from build123d import *

# Parameters (mm, degrees)
TAP_DRILL_FOR_M5_TAP1_D     = 4.1
TAP_DRILL_FOR_M5_TAP1_DEPTH = 5.5
TAP_DRILL_FOR_M5_TAP1_TIP   = 1.231764269
SKETCH5_R                   = 1.75
CUT_EXTRUDE1_DEPTH          = 29.8


with BuildPart() as part:
    # Sketch2 → Revolve4 (revolve)
    with BuildSketch(Plane.XY):
        Polygon((292.362244726, 80.31885353), (304.262244726, 80.31885353), (304.262244726, 80.06885353), (307.762244726, 80.06885353), (307.762244726, 76.84385353), (284.762244726, 76.84385353), (284.762244726, 79.76885353), (287.762244726, 79.76885353), (287.762244726, 79.49385353), (288.762244726, 79.49385353), (288.762244726, 79.82385353), (291.762244726, 79.82385353), (291.762244726, 79.49385353), (292.362244726, 79.49385353), align=None)
    revolve(axis=Axis((307.762244726, 76.84385353, 0), (-1, 0, 0)))

    # Tap Drill for M5 Tap1
    with Locations(Plane(origin=(307.762244726, 0, 0), x_dir=(0, 0, -1), z_dir=(1, 0, 0))):
        with Locations((0, 76.84385353)):
            Hole(TAP_DRILL_FOR_M5_TAP1_D / 2, depth=TAP_DRILL_FOR_M5_TAP1_DEPTH)
            with Locations((0, 0, -(TAP_DRILL_FOR_M5_TAP1_DEPTH + TAP_DRILL_FOR_M5_TAP1_TIP / 2))):  # 118° drill point
                Cone(0, TAP_DRILL_FOR_M5_TAP1_D / 2, TAP_DRILL_FOR_M5_TAP1_TIP, mode=Mode.SUBTRACT)

    # Sketch5 → Cut-Extrude1 (cut)
    with BuildSketch(Plane.ZY.offset(-284.762244726)):
        with Locations((0, 76.84385353)):
            Circle(SKETCH5_R)
    extrude(amount=-CUT_EXTRUDE1_DEPTH, mode=Mode.SUBTRACT)


solid = part.part
Verification items for the finished model (mm, model axes). A direction names the side the tool comes from. Round coordinates to 2 decimals unless told otherwise and drop trailing zeros. Loops run counter-clockwise (first coordinate to the right, second up) from the corner with the lowest first, then second, coordinate; pieces in that order, holes last. Notation, with made-up numbers: (-32.75, -1.5) - (-7.75, -1.5) arc R19 cw to (-7.75, 11.5) - close; hole circle Ø2 at (-7, 34.5). An arc over 180 degrees is marked (long way). Use a Markdown table: item, result. Add a question column.
1. Section check C-C, the plane x = 302.75. Record the boundary of the cut face in (y, z) (3 decimals), plus the area to 3 significant figures.
2. Thickness scan on probe 1 along X at (y, z) = (75.75, 2.5); probe 2 along Y at (x, z) = (289, 0); probe 3 along Y at (x, z) = (305.85, 0). Record the ranges inside material, lowest first. Write a range as [from, to].
3. Section check B-B, the plane x = 286.75. Record the boundary of the cut face in (y, z) (3 decimals).
4. Release check for a two-part mould opening along X. For faces 6 (the face through (298, 74, -2)), 7 (the face through (307.762, 78, 2)), 8 (the face through (288.269, 74.196, -0.117)) record: released by +X, released by -X, zero draft, split by the parting line, or undercut.
5. Gauge pin test, flat ends, axial feed: pin 1 (1 mm diameter, centred on x = 298.5, z = -0.5, fed in from -Y); pin 2 (4 mm diameter, centred on x = 288.5, y = 74, fed in from +Z). Record the tip position at first contact, or that the pin passes through.
6. Access from +Z, -Z, +X, -X, +Y, -Y to the whole of each face (thin tool, end or side, straight path). Record for faces 1 (the face through (284.762, 74.9, 0)), 2 (the face through (286.28, 73.92, -0.13)), 3 (the face through (292.362, 78, 3)), 4 (the face through (306.04, 79.92, -0.97)), 5 (the face through (293.301, 75.135, -0.379)).
Checks:
| question | item | result |
|---|---|---|
| 1 | outline | circle Ø6.95 at (76.844, 0); hole circle Ø4.1 at (76.844, 0) |
| 1 | area | 24.7 mm^2 |
| 2 | probe 1 | x = [284.76, 287.76], [288.76, 291.76], [292.36, 307.76] |
| 2 | probe 2 | y = [73.86, 75.09], [78.59, 79.82] |
| 2 | probe 3 | y = [73.62, 74.79], [78.89, 80.07] |
| 3 | outline | circle Ø5.85 at (76.844, 0); hole circle Ø3.5 at (76.844, 0) |
| 4 | face 6 | zero draft |
| 4 | face 7 | released by +X |
| 4 | face 8 | undercut |
| 5 | pin 1 | stops at y = 73.37 |
| 5 | pin 2 | stops at z = 2.85 |
| 6 | face 1 | +Z, -Z, -X, +Y, -Y |
| 6 | face 2 | -X |
| 6 | face 3 | none |
| 6 | face 4 | +X |
| 6 | face 5 | +X, -X |
